```python
from build123d import *

# Parameters (mm, degrees)
SKETCH1_W           = 30
SKETCH1_H           = 100
SKETCH1_W_2         = 210
SKETCH1_H_2         = 40
BOSS_EXTRUDE1_DEPTH = 8
SKETCH3_R           = 2.1
CUT_EXTRUDE2_DEPTH  = 10
SKETCH2_R           = 2.1
CUT_EXTRUDE3_DEPTH  = 10
SKETCH4_R           = 1.6
CUT_EXTRUDE4_DEPTH  = 10
FILLET1_R           = 5


with BuildPart() as part:
    # Sketch1 → Boss-Extrude1 (new body)
    with BuildSketch(Plane(origin=(0, 0, 0), x_dir=(1, 0, 0), z_dir=(0, 1, 0))):
        Rectangle(SKETCH1_W, SKETCH1_H)
        with Locations((120, 0)):
            Rectangle(SKETCH1_W_2, SKETCH1_H_2)
    extrude(amount=BOSS_EXTRUDE1_DEPTH)

    # Sketch3 → Cut-Extrude2 (cut)
    with BuildSketch(Plane(origin=(0, 8, 0), x_dir=(1, 0, 0), z_dir=(0, 1, 0))):
        with Locations((-9, 0)):
            Circle(SKETCH3_R)
        with Locations((9, 0)):
            Circle(SKETCH3_R)
        with Locations((59, 0)):
            Circle(SKETCH3_R)
        with Locations((109, 0)):
            Circle(SKETCH3_R)
        with Locations((159, 0)):
            Circle(SKETCH3_R)
        with Locations((209, 0)):
            Circle(SKETCH3_R)
    extrude(amount=-CUT_EXTRUDE2_DEPTH, mode=Mode.SUBTRACT)

    # Sketch2 → Cut-Extrude3 (cut)
    with BuildSketch(Plane(origin=(0, 8, 0), x_dir=(1, 0, 0), z_dir=(0, 1, 0))):
        with Locations((-9, -42)):
            Circle(SKETCH2_R)
        with Locations((-9, -18)):
            Circle(SKETCH2_R)
        with Locations((9, -18)):
            Circle(SKETCH2_R)
        with Locations((9, -42)):
            Circle(SKETCH2_R)
        with Locations((9, 42)):
            Circle(SKETCH2_R)
        with Locations((9, 18)):
            Circle(SKETCH2_R)
        with Locations((-9, 18)):
            Circle(SKETCH2_R)
        with Locations((-9, 42)):
            Circle(SKETCH2_R)
    extrude(amount=-CUT_EXTRUDE3_DEPTH, mode=Mode.SUBTRACT)

    # Sketch4 → Cut-Extrude4 (cut)
    with BuildSketch(Plane(origin=(0, 8, 0), x_dir=(1, 0, 0), z_dir=(0, 1, 0))):
        with Locations((59, -15)):
            Circle(SKETCH4_R)
        with Locations((59, 15)):
            Circle(SKETCH4_R)
        with Locations((69, 15)):
            Circle(SKETCH4_R)
        with Locations((69, -15)):
            Circle(SKETCH4_R)
        with Locations((79, 15)):
            Circle(SKETCH4_R)
        with Locations((79, -15)):
            Circle(SKETCH4_R)
        with Locations((89, 15)):
            Circle(SKETCH4_R)
        with Locations((89, -15)):
            Circle(SKETCH4_R)
        with Locations((99, -15)):
            Circle(SKETCH4_R)
        with Locations((99, 15)):
            Circle(SKETCH4_R)
        with Locations((109, -15)):
            Circle(SKETCH4_R)
        with Locations((109, 15)):
            Circle(SKETCH4_R)
        with Locations((119, -15)):
            Circle(SKETCH4_R)
        with Locations((119, 15)):
            Circle(SKETCH4_R)
        with Locations((129, -15)):
            Circle(SKETCH4_R)
        with Locations((129, 15)):
            Circle(SKETCH4_R)
        with Locations((139, -15)):
            Circle(SKETCH4_R)
        with Locations((139, 15)):
            Circle(SKETCH4_R)
        with Locations((149, -15)):
            Circle(SKETCH4_R)
        with Locations((149, 15)):
            Circle(SKETCH4_R)
        with Locations((159, -15)):
            Circle(SKETCH4_R)
        with Locations((159, 15)):
            Circle(SKETCH4_R)
        with Locations((169, -15)):
            Circle(SKETCH4_R)
        with Locations((169, 15)):
            Circle(SKETCH4_R)
        with Locations((179, -15)):
            Circle(SKETCH4_R)
        with Locations((179, 15)):
            Circle(SKETCH4_R)
        with Locations((189, 15)):
            Circle(SKETCH4_R)
        with Locations((189, -15)):
            Circle(SKETCH4_R)
        with Locations((199, 15)):
            Circle(SKETCH4_R)
        with Locations((199, -15)):
            Circle(SKETCH4_R)
        with Locations((209, 15)):
            Circle(SKETCH4_R)
        with Locations((209, -15)):
            Circle(SKETCH4_R)
        with Locations((219, 15)):
            Circle(SKETCH4_R)
        with Locations((219, -15)):
            Circle(SKETCH4_R)
    extrude(amount=-CUT_EXTRUDE4_DEPTH, mode=Mode.SUBTRACT)

    # Fillet1
    fillet1_edges = [part.edges().sort_by_distance(p)[0] for p in [
        (15, 4, -20),
        (225, 4, -20),
        (225, 4, 20),
        (15, 4, 20),
        (15, 4, 50),
        (-15, 4, 50),
        (-15, 4, -50),
        (15, 4, -50),
    ]]
    fillet(fillet1_edges, radius=FILLET1_R)


solid = part.part
```
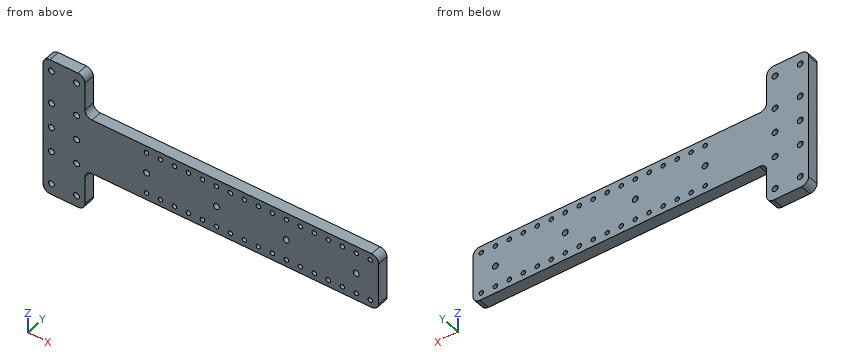
The model under review builds one solid part; all positions refer to its coordinate system, in mm. Coordinates: 2 decimals unless noted, no trailing zeros. Order: outer loops, then holes, each group sorted by start corner. A loop starts at its lowest first (then second) coordinate and runs counter-clockwise, first axis right, second up. Notation, with made-up numbers: (12.25, 10.25) -> (20.25, 10.25) arc R21 cw to (20.25, 43.25) -> close; hole circle Ø2 at (76, 87.5). An arc over 180 degrees is marked (long way). Answer in a Markdown table with one row per item. Add a question column.
Item 1: We need section C-C on x = 74. Write out the cut boundary in (y, z).
Item 2: We need section A-A on z = -42. Write out the cut boundary in (x, y).
Item 3: We need section B-B on y = 2. Give the number of separate pieces and of enclosed holes in the cut face, plus the area to 3 significant figures.
Item 4: To check wall thickness, follow probe 1 along Z at (x, y) = (139, 4); probe 2 along X at (y, z) = (3.75, -42); probe 3 along Z at (x, y) = (-9, 2.5). State the ranges of each line that lie inside material, in increasing order.
Item 5: Clearance check with a flat-ended pin moving along its axis: pin 1 (4 mm diameter, centred on x = 128, y = 2, fed in from -Z). State where the tip first meets the part, or that it passes through.
Final values:
| question | item | result |
|---|---|---|
| 1 | outline | (0, -20) -> (8, -20) -> (8, 20) -> (0, 20) -> close |
| 2 | outline | (-15, 0) -> (-11.1, 0) -> (-11.1, 8) -> (-15, 8) -> close; (-6.9, 0) -> (6.9, 0) -> (6.9, 8) -> (-6.9, 8) -> close; (11.1, 0) -> (15, 0) -> (15, 8) -> (11.1, 8) -> close |
| 3 | separate pieces | 1 |
| 3 | enclosed holes | 48 |
| 3 | area | 10,900 mm2 |
| 4 | probe 1 | z = -20 to -16.6, -13.4 to 13.4, 16.6 to 20 |
| 4 | probe 2 | x = -15 to -11.1, -6.9 to 6.9, 11.1 to 15 |
| 4 | probe 3 | z = -50 to -44.1, -39.9 to -20.1, -15.9 to -2.1, 2.1 to 15.9, 20.1 to 39.9, 44.1 to 50 |
| 5 | pin 1 | stops at z = -20 |
